The drawing under review shows one solid part. Ordinate dimensions are in mm from its lowest x, y, z. A direction names the side the tool comes from. Give positions to 0.01 mm unless a question says otherwise; leave off trailing zeros. Loops run counter-clockwise (first coordinate to the right, second up) from the corner with the lowest first, then second, coordinate; pieces in that order, holes last. Notation, with made-up numbers: (-23, 80.5) - (31, 80.5) arc R23 ccw to (31, 116.5) - close; hole circle Ø3 at (19, 88). An arc over 180 degrees is marked (long way). Answer as CSV lines item,"result".
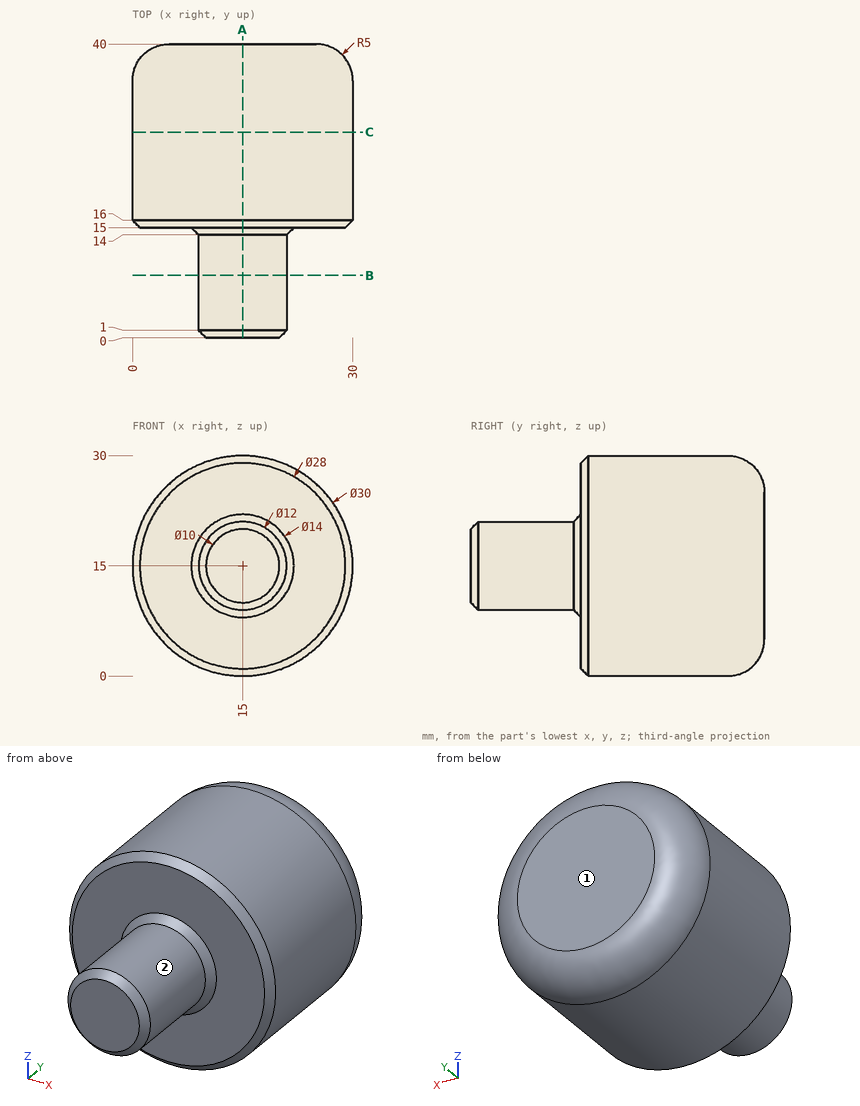
1) Consider section B-B on y = 8.5. Write out the cut boundary in (x, z).
From the geometry:
outline,"circle Ø12 at (15, 15)"
2) Insertion check: P1, Ø1, axis at y = 19, z = 23, coming from the -X side; P2, Ø5, axis at x = 11.5, z = 6, coming from the -Y side; P3, Ø10, axis at y = 11, z = 24.5, coming from the -X side. Each pin has a flat end and moves straight along its axis. Give the tip position at first contact, or say it passes through.
From the geometry:
P1,"stops at x = 2.01"
P2,"stops at y = 15"
P3,"stops at x = 2.48"
3) Consider section C-C on y = 28. Write out the cut boundary in (x, z).
From the geometry:
outline,"circle Ø30 at (15, 15)"
4) Machinability: for the marked faces 1 and 2, which of the approach directions +Z, -Z, +X, -X, +Y, -Y give a long, thin tool a straight path to every point of the face, cutting with its end or side? Answer none if there is none.
From the geometry:
face 1,"+Z, -Z, +X, -X, +Y"
face 2,"-Y"
5) Wall thickness on line 1 (Y direction, x = 13.75, z = 23); line 2 (X direction, y = 19.5, z = 14.5); line 3 (Y direction, x = 1.75, z = 17): over which ranges is each line inside the solid? List them lowest first. Write a range as from..to.
From the geometry:
line 1,"y = 15..40"
line 2,"x = 0.01..29.99"
line 3,"y = 15..38.67"
6) Consider section A-A on x = 15. Write out the cut boundary in (y, z).
From the geometry:
outline,"(0, 10) - (1, 9) - (14, 9) - (15, 8) - (15, 1) - (16, 0) - (35, 0) arc R5 ccw to (40, 5) - (40, 25) arc R5 ccw to (35, 30) - (16, 30) - (15, 29) - (15, 22) - (14, 21) - (1, 21) - (0, 20) - close"
